Work out the finished part from the listing and answer in its coordinate system (mm). Coordinates: 2 decimals unless noted, no trailing zeros. Order: outer loops, then holes, each group sorted by start corner. A loop starts at its lowest first (then second) coordinate and runs counter-clockwise, first axis right, second up. Notation, with made-up numbers: (2.25, 77.5) -> (56.25, 77.5) arc R26 ccw to (56.25, 105.5) -> close; hole circle Ø5 at (13.25, 5.5). An arc over 180 degrees is marked (long way). Answer as CSV lines item,"result". Start each with the question number.
Item 1: Section B-B (z = 8) is taken. Write down the section's boundary in (x, y), then the cut area to 3 significant figures.
Item 2: Straight lines are drawn through the part: L1, parallel to X at y = 3.6, z = -17 (3 decimals); L2, parallel to X at y = 2.1, z = -60. For each, find the intervals that lie inside material, in ascending order.
Item 3: Section A-A (x = 37) is taken. Write down the section's boundary in (y, z).
```python
from build123d import *

# Parameters (mm, degrees)
SKETCH1_W           = 140
SKETCH1_H           = 140
BOSS_EXTRUDE1_DEPTH = 5
SKETCH2_R           = 1.5
CUT_EXTRUDE1_DEPTH  = 5
CUT_EXTRUDE2_DEPTH  = 5
SKETCH6_R           = 1.5
CUT_EXTRUDE4_DEPTH  = 5


with BuildPart() as part:
    # Sketch1 → Boss-Extrude1 (new body)
    with BuildSketch(Plane(origin=(0, 0, 0), x_dir=(1, 0, 0), z_dir=(0, 1, 0))):
        Rectangle(SKETCH1_W, SKETCH1_H)
    extrude(amount=BOSS_EXTRUDE1_DEPTH)

    # Sketch2 → Cut-Extrude1 (cut)
    with BuildSketch(Plane.XZ):
        with Locations(Location((24.505, -17.005, 0), (0, 0, 270))):
            Circle(SKETCH2_R)
        with Locations(Location((-17.005, -24.505, 0), (0, 0, 270))):
            Circle(SKETCH2_R)
        with Locations(Location((-24.505, 17.005, 0), (0, 0, 270))):
            Circle(SKETCH2_R)
        with Locations(Location((17.005, 24.505, 0), (0, 0, 270))):
            Circle(SKETCH2_R)
    extrude(amount=-CUT_EXTRUDE1_DEPTH, mode=Mode.SUBTRACT)

    # Sketch4 → Cut-Extrude2 (cut)
    with BuildSketch(Plane(origin=(0, 5, 0), x_dir=(1, 0, 0), z_dir=(0, 1, 0))):
        Polygon((-14, 42), (14, 42), (14, 14), (42, 14), (42, -14), (14, -14), (14, -42), (-14, -42), (-14, -14), (-42, -14), (-42, 14), (-14, 14), align=None)
    extrude(amount=-CUT_EXTRUDE2_DEPTH, mode=Mode.SUBTRACT)

    # Sketch6 → Cut-Extrude4 (cut)
    with BuildSketch(Plane(origin=(0, 5, 0), x_dir=(1, 0, 0), z_dir=(0, 1, 0))):
        with Locations(Location((-60, 60, 0), (0, 0, 270))):
            Circle(SKETCH6_R)
        with Locations(Location((60, 60, 0), (0, 0, 270))):
            Circle(SKETCH6_R)
        with Locations(Location((60, -60, 0), (0, 0, 270))):
            Circle(SKETCH6_R)
        with Locations(Location((-60, -60, 0), (0, 0, 270))):
            Circle(SKETCH6_R)
    extrude(amount=-CUT_EXTRUDE4_DEPTH, mode=Mode.SUBTRACT)


solid = part.part
```
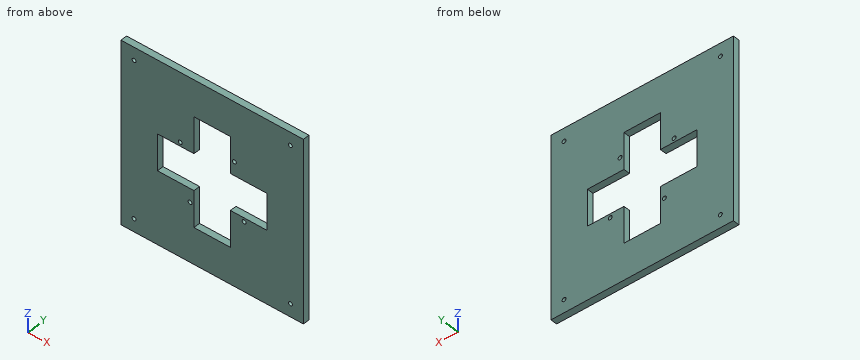
Checked values:
1,outline,"(-70, 0) -> (-42, 0) -> (-42, 5) -> (-70, 5) -> close; (42, 0) -> (70, 0) -> (70, 5) -> (42, 5) -> close"
1,area,"280 mm^2"
2,L1,"x = -70 to -14, 14 to 23.005, 26.005 to 70"
2,L2,"x = -70 to -61.5, -58.5 to 58.5, 61.5 to 70"
3,outline,"(0, -70) -> (5, -70) -> (5, -14) -> (0, -14) -> close; (0, 14) -> (5, 14) -> (5, 70) -> (0, 70) -> close"
